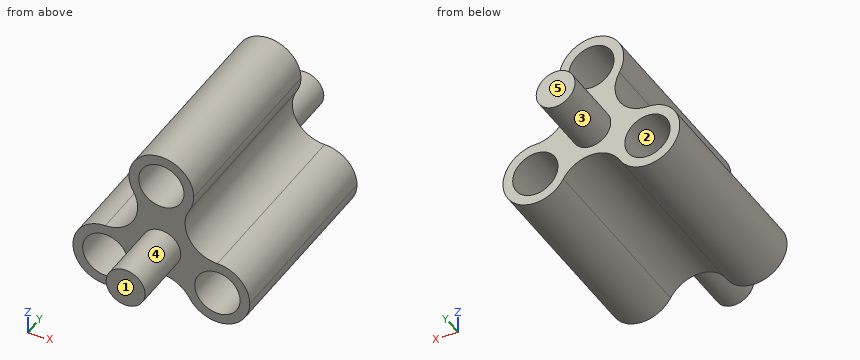
```python
from build123d import *

# Parameters (mm, degrees)
F0_R          = 3.5
F1_DEPTH      = 30
F2_R          = 3
F3_DEPTH      = 40
F3_DEPTH_BACK = 10


# Not quite as in the source:
# - ends of sketch curves that miss each other by under 0.0002 mm in the source are joined


with BuildPart() as f1:
    # F0 (on Front) → F1 (new body)
    with BuildSketch(Plane.XZ):
        with BuildLine():
            ThreePointArc((-4.3301281481, 8.0578746702), (-6.557e-07, 5.5578757428), (4.330125744, 8.057876563))
            ThreePointArc((4.330125744, 8.057876563), (4.8296291409, 9.2637805524), (5, 10.5578757428))
            ThreePointArc((5, 10.5578757428), (-1.2940954014, 15.3875048271), (-4.3301281481, 8.0578746702))
        make_face()
        with Locations((0, 10.5578757428)):
            Circle(F0_R, mode=Mode.SUBTRACT)
        with BuildLine():
            ThreePointArc((8.6602543293, 0.557875869), (4.3301271646, 3.0578757428), (4.3301270553, 8.0578758059))
            ThreePointArc((4.3301270553, 8.0578758059), (-6.557e-07, 5.5578757428), (-4.3301281481, 8.0578746702))
            ThreePointArc((-4.3301281481, 8.0578746702), (-4.330127711, 3.0578747964), (-8.6602543293, 0.5578743547))
            ThreePointArc((-8.6602543293, 0.5578743547), (-5.1247199995, -0.9065915075), (-3.6602536736, -4.4421256453))
            ThreePointArc((-3.6602536736, -4.4421256453), (-3.8306244761, -5.7362206245), (-4.3301263997, -6.9421252036))
            ThreePointArc((-4.3301263997, -6.9421252036), (4.371e-07, -4.442124762), (4.330127711, -6.9421244465))
            ThreePointArc((4.330127711, -6.9421244465), (4.3301273832, -1.9421243834), (8.6602543293, 0.557875869))
        make_face()
        with BuildLine():
            ThreePointArc((13.6602545478, -4.442124131), (12.1957883765, -0.9065901478), (8.6602543293, 0.557875869))
            ThreePointArc((8.6602543293, 0.557875869), (4.3301273832, -1.9421243834), (4.330127711, -6.9421244465))
            ThreePointArc((4.330127711, -6.9421244465), (9.9543499492, -9.2717532153), (13.6602545478, -4.442124131))
        make_face()
        with Locations((8.6602545478, -4.442124131)):
            Circle(F0_R, mode=Mode.SUBTRACT)
        with BuildLine():
            ThreePointArc((-3.6602536736, -4.4421256453), (-5.1247199995, -0.9065915075), (-8.6602543293, 0.5578743547))
            ThreePointArc((-8.6602543293, 0.5578743547), (-12.9903804011, -6.94212615), (-4.3301263997, -6.9421252036))
            ThreePointArc((-4.3301263997, -6.9421252036), (-3.8306244761, -5.7362206245), (-3.6602536736, -4.4421256453))
        make_face()
        with Locations((-8.6602536736, -4.4421256453)):
            Circle(F0_R, mode=Mode.SUBTRACT)
    extrude(amount=F1_DEPTH)

    # F2 (on Front) → F3 (join, two sides)
    with BuildSketch(Plane.XZ) as f3_sk:
        Circle(F2_R)
    extrude(amount=F3_DEPTH)
    extrude(f3_sk.sketch, amount=-F3_DEPTH_BACK)


solid = f1.part
```
The model under review builds one solid part; all positions refer to its coordinate system, in mm. Face numbers are marked on the shaded views. A direction names the side the tool comes from. Round coordinates to 2 decimals unless told otherwise and drop trailing zeros. Write each loop counter-clockwise with the first axis right and the second up, starting at its lowest first coordinate (ties: lowest second). Pieces come first, ordered by that corner, then holes. Notation, with made-up numbers: (-3.75, -9) - (37.25, -9) arc R23 ccw to (37.25, 28) - close; hole circle Ø3 at (3.25, -30.5). An arc over 180 degrees is marked (long way). One line per question, with ' | ' between items.
Item 1: For P1, Ø8, axis at x = 0, z = 10.56, coming from the -Y side; P2, Ø12, axis at y = -3, z = 4.5, coming from the +X side; P3, Ø3, axis at x = 5.5, y = -11.5, coming from the -Z side; P4, Ø5.5, axis at x = -8.66, z = -4.44, coming from the +Y side, all flat-tipped, find the tip position at first contact; note any pin that passes through.
Resolved:
P1: stops at y = -30 | P2: stops at x = 12.7 | P3: stops at z = -9.16 | P4: passes through
Item 2: The part is to be moulded in two halves that separate along X. For the marked faces 1, 2 and 3, say which applies: pulls with the +X half, pulls with the -X half, needs draft (parallel to the pull), parting line crosses it, or undercut.
Resolved:
face 1: needs draft | face 2: undercut | face 3: parting line crosses it
Item 3: Add section C-C, the plane z = 2. Give the boundary of the cut face in (x, y), then the cut area to 3 significant figures.
Resolved:
outline: (-5.15, -30) - (-2.24, -30) - (-2.24, -40) - (2.24, -40) - (2.24, -30) - (5.15, -30) - (5.15, 0) - (2.24, 0) - (2.24, 10) - (-2.24, 10) - (-2.24, 0) - (-5.15, 0) - close | area: 398 mm2
Item 4: Add section A-A, the plane x = 0. Give the boundary of the cut face in (y, z).
Resolved:
outline: (-40, -3) - (-30, -3) - (-30, -4.44) - (0, -4.44) - (0, -3) - (10, -3) - (10, 3) - (0, 3) - (0, 7.06) - (-30, 7.06) - (-30, 3) - (-40, 3) - close; (-30, 14.06) - (0, 14.06) - (0, 15.56) - (-30, 15.56) - close
Item 5: To check wall thickness, follow probe 1 along X at (y, z) = (-2, -6.5); probe 2 along X at (y, z) = (-27.5, -7.25); probe 3 along X at (y, z) = (-17, -8). State the ranges of each line that lie inside material, in increasing order.
Resolved:
probe 1: x = -13.22 to -11.49, -5.83 to -4.04, 4.04 to 5.83, 11.49 to 13.22 | probe 2: x = -12.8 to -10.75, -6.57 to -4.52, 4.52 to 6.57, 10.75 to 12.8 | probe 3: x = -12.17 to -5.15, 5.15 to 12.17
Item 6: For the marked faces 4 and 5, list the 3-axis set-ups (+Z, -Z, +X, -X, +Y, -Y) from which the entire face can be reached by the end or side of a thin tool; tool diameter is ignored.
Resolved:
face 4: -Y | face 5: +Z, -Z, +X, -X, +Y
Item 7: Add section D-D, the plane z = -6. Give the boundary of the cut face in (x, y).
Resolved:
outline: (-13.41, -30) - (-11.79, -30) - (-11.79, 0) - (-13.41, 0) - close; (-5.53, -30) - (-3.63, -30) - (-3.63, 0) - (-5.53, 0) - close; (3.63, -30) - (5.53, -30) - (5.53, 0) - (3.63, 0) - close; (11.79, -30) - (13.41, -30) - (13.41, 0) - (11.79, 0) - close
Item 8: Add section B-B, the plane y = -13. Give the boundary of the cut face in (x, z).
Resolved:
outline: (-8.66, 0.56) arc R5 ccw (long way) to (-4.33, -6.94) arc R5 cw to (4.33, -6.94) arc R5 ccw (long way) to (8.66, 0.56) arc R5 cw to (4.33, 8.06) arc R5 ccw to (5, 10.56) arc R5 ccw (long way) to (-4.33, 8.06) arc R5 cw to start; hole circle Ø7 at (-8.66, -4.44); hole circle Ø7 at (0, 10.56); hole circle Ø7 at (8.66, -4.44)
